Here's how the part is built. I have some questions about the finished solid (model axes, mm). Round coordinates to 2 decimals unless told otherwise and drop trailing zeros. Order: outer loops, then holes, each group sorted by start corner. A loop starts at its lowest first (then second) coordinate and runs counter-clockwise, first axis right, second up. Notation, with made-up numbers: (33.5, 81) -> (88.5, 81) arc R13 ccw to (88.5, 100) -> close; hole circle Ø10 at (70, 8). An arc over 180 degrees is marked (long way). Use a Markdown table: item, result. Add a question column.
from build123d import *


with BuildPart() as part:
    # ｽｹｯﾁ1 → 回転1 (revolve)
    with BuildSketch(Plane.XY, mode=Mode.PRIVATE) as revolve_1_sk:
        with BuildLine():
            Line((1.25, 13.149), (1.25, 10))
            Line((1.25, 10), (14.25, 10))
            ThreePointArc((14.25, 10), (14.957106781, 10.292893219), (15.25, 11))
            Line((15.25, 11), (15.25, 16.75))
            Line((15.25, 16.75), (13.131049, 16.75))
            Line((13.131049, 16.75), (12.570253493, 16.580029771))
            Line((12.570253493, 16.580029771), (12.9498679, 14.104804989))
            Line((12.9498679, 14.104804989), (3.329373052, 13.418096908))
            Line((3.329373052, 13.418096908), (3.276447429, 13.763191322))
            Line((3.276447429, 13.763191322), (1.25, 13.149))
        make_face()
    revolve(revolve_1_sk.sketch.rotate(Axis((1.25, 0, 0), (1, 0, 0)), 270), axis=Axis((1.25, 0, 0), (1, 0, 0)))


solid = part.part
(1) I'm going to push flat-ended pins straight in: P1, Ø12, axis at y = 0, z = 0, coming from the +X side; P2, Ø6, axis at x = 10.5, y = -6, coming from the -Z side; P3, Ø3, axis at x = 12, y = -4.5, coming from the +Z side; P4, Ø4, axis at x = 13.5, z = -12.5, coming from the -Y side. Where does each tip first touch, or does it pass through?
(2) Please list where these lines run through material, in increasing order: probe 1 along Y at (x, z) = (12.25, -2); probe 2 along Z at (x, y) = (7.25, 4); probe 3 along Y at (x, z) = (8.75, 0). Write a range as from..to.
(3) I want a section at A-A on z = 0. List the corners of the cut face in (x, y) for me, and give its area (3 significant figures).
(4) If we mould it in two halves opening along X, with no side actions, what happens to faces 1 (the flat face through (15.25, -3, 11)), 2 (the conical face through (7.003, -13.355, 2.966)), 3 (the flat face through (1.25, 10, 2)), 4 (the cylindrical face through (7.84, -9.76, 2.17))? For each: pulls with the +X half, pulls with the -X half, needs draft (parallel to the pull), parting line crosses it, or undercut.
(5) I want a section at D-D on x = 7.5. List the corners of the cut face in (y, z) for me, and give its area (3 significant figures).
(6) I want a section at B-B on x = 13.75. List the corners of the cut face in (y, z) for me.
Output:
| question | item | result |
|---|---|---|
| 1 | P1 | through |
| 1 | P2 | z = -16.14 |
| 1 | P3 | z = 16.38 |
| 1 | P4 | y = -13.05 |
| 2 | probe 1 | -13.91..-9.8, 9.8..13.91 |
| 2 | probe 2 | -13.1..-9.17, 9.17..13.1 |
| 2 | probe 3 | -13.81..-10, 10..13.81 |
| 3 | outline | (1.25, -13.15) -> (3.28, -13.76) -> (3.33, -13.42) -> (12.95, -14.1) -> (12.57, -16.58) -> (13.13, -16.75) -> (15.25, -16.75) -> (15.25, -11) arc R1 ccw to (14.25, -10) -> (1.25, -10) -> close; (1.25, 10) -> (14.25, 10) arc R1 ccw to (15.25, 11) -> (15.25, 16.75) -> (13.13, 16.75) -> (12.57, 16.58) -> (12.95, 14.1) -> (3.33, 13.42) -> (3.28, 13.76) -> (1.25, 13.15) -> close |
| 3 | area | 118 mm² |
| 4 | face 1 | pulls with the +X half |
| 4 | face 2 | undercut |
| 4 | face 3 | pulls with the -X half |
| 4 | face 4 | needs draft |
| 5 | outline | circle Ø27.43 at (0, 0); hole circle Ø20 at (0, 0) |
| 5 | area | 277 mm² |
| 6 | outline | circle Ø33.5 at (0, 0); hole circle Ø20 at (0, 0) |
